Job drawing, mm, ordinate dimensions from the low corner. One solid piece. A direction names the side the tool comes from. Round coordinates to 2 decimals unless told otherwise and drop trailing zeros. Loops run counter-clockwise (first coordinate to the right, second up) from the corner with the lowest first, then second, coordinate; pieces in that order, holes last. Notation, with made-up numbers: M -5.75,-8 L 41.25,-8 A35 cw 41.25,30 Z; hole C 24.5,53 d8. An arc over 180 degrees is marked long. Use one line per item in the form item = value. Start each with the question number.
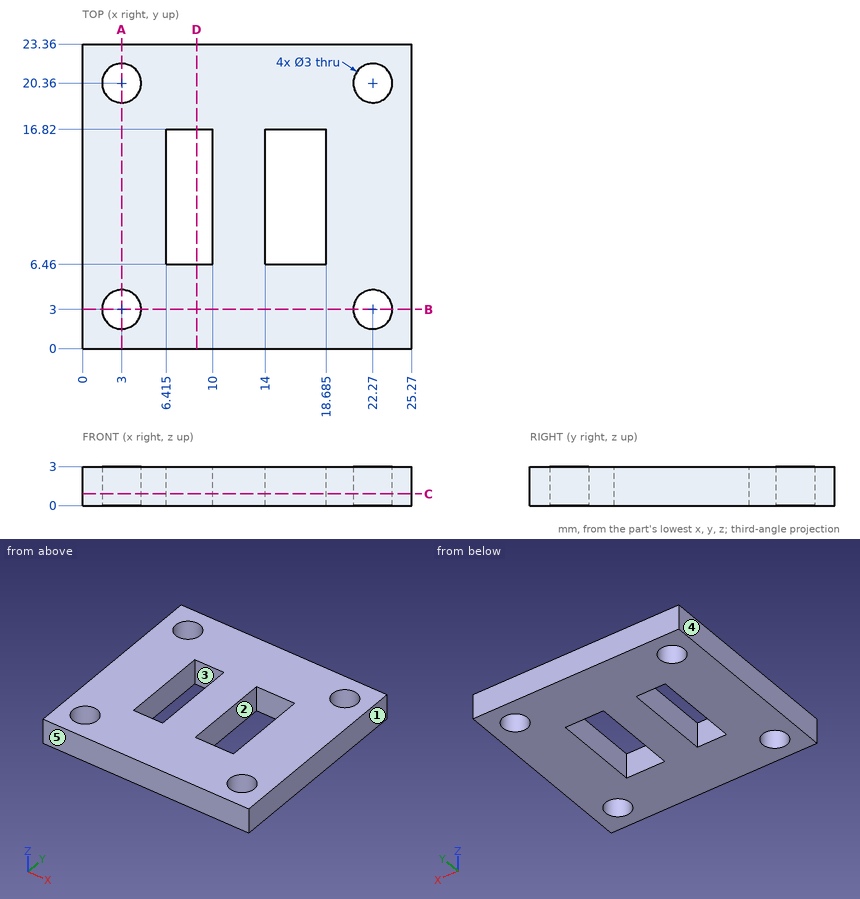
Q1. Saw through at C-C (z = 0.9). Give the cut face in (x, y) (3 decimals).
Q2. Drop flat-ended pins along their axis: P1, Ø2.5, axis at x = 22.27, y = 3, coming from the +Z side; P2, Ø5, axis at x = 7.5, y = 9, coming from the -Z side. Give the stop position or say it passes through.
Q3. Saw through at A-A (x = 3). Give the cut face in (y, z).
Q4. Saw through at B-B (y = 3). Give the cut face in (x, z), and give its area (3 significant figures).
Q5. Wall check: probe 1 along X at (y, z) = (14, 0.3) (3 decimals); probe 2 along Y at (x, z) = (3, 1.05); probe 3 along X at (y, z) = (4, 0.75). Give the ranges that are in metal, low to high.
Q6. Saw through at D-D (x = 8.75). Give the cut face in (y, z).
Q7. Pull direction X, two halves, no side cores. Call the marked faces 3, 4 and 5: pulls with the +X half, pulls with the -X half, needs draft (parallel to the pull), parting line crosses it, or undercut.
Q8. Tool access for the marked faces 1 and 2: list every direction of +Z, -Z, +X, -X, +Y, -Y with a clear straight run to the whole face (end or side of a thin tool).
Filled in:
q1.outline = M 0,0 L 25.27,0 L 25.27,23.36 L 0,23.36 Z; hole C 3,3 d3; hole C 3,20.36 d3; hole M 6.415,6.46 L 10,6.46 L 10,16.82 L 6.415,16.82 Z; hole M 14,6.46 L 18.685,6.46 L 18.685,16.82 L 14,16.82 Z; hole C 22.27,3 d3; hole C 22.27,20.36 d3
q2.P1 = through
q2.P2 = 0
q3.outline = M 0,0 L 1.5,0 L 1.5,3 L 0,3 Z; M 4.5,0 L 18.86,0 L 18.86,3 L 4.5,3 Z; M 21.86,0 L 23.36,0 L 23.36,3 L 21.86,3 Z
q4.outline = M 0,0 L 1.5,0 L 1.5,3 L 0,3 Z; M 4.5,0 L 20.77,0 L 20.77,3 L 4.5,3 Z; M 23.77,0 L 25.27,0 L 25.27,3 L 23.77,3 Z
q4.area = 57.8 mm²
q5.probe_1 = 0 to 6.415, 10 to 14, 18.685 to 25.27
q5.probe_2 = 0 to 1.5, 4.5 to 18.86, 21.86 to 23.36
q5.probe_3 = 0 to 1.88, 4.12 to 21.15, 23.39 to 25.27
q6.outline = M 0,0 L 6.46,0 L 6.46,3 L 0,3 Z; M 16.82,0 L 23.36,0 L 23.36,3 L 16.82,3 Z
q7.face_3 = undercut
q7.face_4 = pulls with the -X half
q7.face_5 = needs draft
q8.face_1 = +Z, -Z, +X, +Y, -Y
q8.face_2 = +Z, -Z
